from build123d import *

# Parameters (mm, degrees)
SKETCH1_R             = 35
SKETCH1_R_2           = 25
BOSS_EXTRUDE1_DEPTH   = 25
BOSS_EXTRUDE1_2_DEPTH = 25
BOSS_EXTRUDE3_DEPTH   = 12
FILLET1_R             = 44
FILLET2_R             = 60
SKETCH3_R             = 6
BOSS_EXTRUDE4_DEPTH   = 30
CUT_EXTRUDE1_DEPTH    = 6


with BuildPart() as part:
    # Sketch1 → Boss-Extrude1 (new, symmetric)
    with BuildSketch(Plane.XY):
        Circle(SKETCH1_R)
        Circle(SKETCH1_R_2, mode=Mode.SUBTRACT)
    extrude(amount=BOSS_EXTRUDE1_DEPTH, both=True)



with BuildPart() as body_2:
    # Sketch1 → Boss-Extrude1 2 (new, symmetric)
    with BuildSketch(Plane.XY):
        with BuildLine():
            Line((400, 50), (400, 60))
            ThreePointArc((400, 60), (340, 0), (400, -60))
            Line((400, -60), (400, -50))
            ThreePointArc((400, -50), (350, 0), (400, 50))
        make_face()
    extrude(amount=BOSS_EXTRUDE1_2_DEPTH, both=True)


with BuildPart() as part_1:
    add(part.part)

    add(body_2.part)  # Boss-Extrude3 merges body 2
    # Sketch2 → Boss-Extrude3 (add, symmetric)
    with BuildSketch(Plane.XY):
        with BuildLine():
            Line((35, 25), (340, 25))
            Line((340, 25), (356, 60))
            Line((356, 60), (400, 60))
            ThreePointArc((400, 60), (340, 0), (400, -60))
            Line((400, -60), (356, -60))
            Line((356, -60), (340, -25))
            Line((340, -25), (35, -25))
            Line((35, -25), (24.494897428, -25))
            ThreePointArc((24.494897428, -25), (35, 0), (24.494897428, 25))
            Line((24.494897428, 25), (35, 25))
        make_face()
    extrude(amount=BOSS_EXTRUDE3_DEPTH, both=True)

    # Fillet1
    fillet1_edges = [part_1.edges().sort_by_distance(p)[0] for p in [
        (24.494897428, 25, 0),
        (24.494897428, -25, 0),
    ]]
    fillet(fillet1_edges, radius=FILLET1_R)

    # Fillet2
    # the kernel refuses this fillet: 60 mm, written as the material it adds along each edge
    with BuildSketch(Plane(origin=(340, -25, 12), x_dir=(-1, 0, 0), z_dir=(0, 0, -1))) as fillet2_piece_1_section:
        with BuildLine():
            CenterArc((FILLET2_R * 0.642393223137, -FILLET2_R), FILLET2_R, 90, 65.432828679)
            Line((-FILLET2_R * 0.267081252449, -FILLET2_R * 0.584240239732), (0, 0))
            Line((0, 0), (FILLET2_R * 0.642393223137, 0))
        make_face()
    fillet2_piece_1 = extrude(amount=24, mode=Mode.PRIVATE)
    fillet2_piece_1 = split(fillet2_piece_1, bisect_by=Plane(origin=(335.089440869, -60, 0), z_dir=(0, 1, 0)), keep=Keep.TOP, mode=Mode.PRIVATE)
    add(fillet2_piece_1)
    with BuildSketch(Plane(origin=(340, 25, 12), x_dir=(0.41575976026779565, 0.9094744755857994, 0), z_dir=(0, 0, -1))) as fillet2_piece_2_section:
        with BuildLine():
            CenterArc((FILLET2_R * 0.642393223137, -FILLET2_R), FILLET2_R, 90, 65.432828679)
            Line((-FILLET2_R * 0.267081252449, -FILLET2_R * 0.584240239732), (0, 0))
            Line((0, 0), (FILLET2_R * 0.642393223137, 0))
        make_face()
    fillet2_piece_2 = extrude(amount=24, mode=Mode.PRIVATE)
    fillet2_piece_2 = split(fillet2_piece_2, bisect_by=Plane(origin=(335.089440869, 60, 0), z_dir=(0, -1, 0)), keep=Keep.TOP, mode=Mode.PRIVATE)
    add(fillet2_piece_2)

    # Sketch3 → Boss-Extrude4 (add)
    with BuildSketch(Plane(origin=(400, 0, 0), x_dir=(0, 0, -1), z_dir=(1, 0, 0))):
        with BuildLine():
            Line((-12, 78), (-12, 60))
            Line((-12, 60), (12, 60))
            Line((12, 60), (12, 78))
            ThreePointArc((12, 78), (0, 90), (-12, 78))
        make_face()
        with Locations((0, 78)):
            Circle(SKETCH3_R, mode=Mode.SUBTRACT)
    boss_extrude4 = extrude(amount=-BOSS_EXTRUDE4_DEPTH)

    # Mirror1: Boss-Extrude4 across plane
    add(boss_extrude4.mirror(Plane.ZX))

    # Sketch4 → Cut-Extrude1 (cut)
    with BuildSketch(Plane.XY.offset(12)):
        with BuildLine():
            Line((280, -14), (80, -14))
            ThreePointArc((80, -14), (66, 0), (80, 14))
            Line((80, 14), (280, 14))
            ThreePointArc((280, 14), (294, 0), (280, -14))
        make_face()
    cut_extrude1 = extrude(amount=-CUT_EXTRUDE1_DEPTH, mode=Mode.SUBTRACT)

    # Mirror2: Cut-Extrude1 across plane
    add(cut_extrude1.mirror(Plane.XY), mode=Mode.SUBTRACT)


solid = part_1.part
Can you work these out from the model? Positions are in its coordinate system, mm. A direction names the side the tool comes from. Coordinates: 2 decimals unless noted, no trailing zeros. Loops run counter-clockwise (first coordinate to the right, second up) from the corner with the lowest first, then second, coordinate; pieces in that order, holes last. Notation, with made-up numbers: (-10, -14) - (4, -14) arc R20 cw to (4, 16) - close; hole circle Ø11 at (70, 24). An arc over 180 degrees is marked (long way). Put each result on its own line as item: value. Start each with the question number.
Item 1: Suppose I cut it at A-A (x = 0). Please give me the cut outline in (y, z), and give its area (3 significant figures).
Item 2: Suppose I cut it at D-D (z = -20). Please give me the cut outline in (x, y).
Item 3: Which directions (+Z, -Z, +X, -X, +Y, -Y) give clear straight access to the entire face, cutting with the end or side of a thin tool? Please do faces 5 (the face through (27.25, -26.455, 0.168)), 6 (the face through (350, -9, 25)), 7 (the face through (334.26, 34.76, 0.17)), 8 (the face through (294, 0, 9)).
Item 4: If I drill on line 1 along Y through (x, z) = (0, 15.5); line 2 along X through (y, z) = (5, -10); line 3 along Y through (x, z) = (149, 7), over which ranges is the centre line in solid material (lowest first)?
Item 5: If we mould it in two halves opening along X, with no side actions, what happens to faces 1 (the face through (400, -66, 0)), 2 (the face through (363, -60, 0)), 3 (the face through (182, 0, -6)), 4 (the face through (370, 72, 3))? For each: +X half, -X half, draft (parallel to the pull), parting line (faces both ways), or undercut.
Item 6: For pin 1 (1 mm diameter, centred on y = -29.5, z = -19, fed in from +X); pin 2 (4 mm diameter, centred on x = 363, z = 2.5, fed in from +Y); pin 3 (10 mm diameter, centred on x = 271.5, y = 8, fed in from +Z), each with a flat end and sliding along its axis, tell me the tip position at first contact or that it passes through.
Item 7: Suppose I cut it at C-C (z = 0). Please give me the cut outline in (x, y).
Item 8: Suppose I cut it at B-B (y = 0). Please give me the cut outline in (x, z), and give its area (3 significant figures).
Here are the results:
1. outline: (-35, -25) - (-25, -25) - (-25, 25) - (-35, 25) - close; (25, -25) - (35, -25) - (35, 25) - (25, 25) - close
1. area: 1,000 mm²
2. outline: circle Ø70 at (0, 0); (400, -60) - (400, -50) arc R50 cw to (400, 50) - (400, 60) arc R60 ccw to start; hole circle Ø50 at (0, 0)
3. face 5: +Z, -Z, -Y
3. face 6: +Z, +X, -X, +Y, -Y
3. face 7: +Z, -Z, +Y
3. face 8: +Z
4. line 1: -35 to -25, 25 to 35
4. line 2: -34.64 to -24.49, 24.49 to 66.92, 293.08 to 350.25
4. line 3: -25 to -14, 14 to 25
5. face 1: +X half
5. face 2: draft
5. face 3: undercut
5. face 4: -X half
6. pin 1: x = 360
6. pin 2: y = 60
6. pin 3: z = 6
7. outline: (17.04, -30.57) arc R44 cw to (38.47, -25) - (301.46, -25) arc R60 cw to (356, -60) - (370, -60) - (370, -72) - (400, -72) - (400, -50) arc R50 cw to (400, 50) - (400, 72) - (370, 72) - (370, 60) - (356, 60) arc R60 cw to (301.46, 25) - (38.47, 25) arc R44 cw to (17.04, 30.57) arc R35 ccw (long way) to start; (370, -90) - (400, -90) - (400, -84) - (370, -84) - close; (370, 84) - (400, 84) - (400, 90) - (370, 90) - close; hole circle Ø50 at (0, 0)
8. outline: (-35, -25) - (-25, -25) - (-25, 25) - (-35, 25) - close; (25, -25) - (35, -25) - (35, -12) - (66, -12) - (66, -6) - (294, -6) - (294, -12) - (340, -12) - (340, -25) - (350, -25) - (350, 25) - (340, 25) - (340, 12) - (294, 12) - (294, 6) - (66, 6) - (66, 12) - (35, 12) - (35, 25) - (25, 25) - close
8. area: 6,080 mm²
